Job drawing, mm, ordinate dimensions from the low corner. One solid piece. A direction names the side the tool comes from. Round coordinates to 2 decimals unless told otherwise and drop trailing zeros. Loops run counter-clockwise (first coordinate to the right, second up) from the corner with the lowest first, then second, coordinate; pieces in that order, holes last. Notation, with made-up numbers: M 15,-24.75 L 37,-24.75 A28 cw 37,-4.75 Z; hole C -15.5,72.25 d4. An arc over 180 degrees is marked long. Use a Markdown table: item, result. Add a question column.
(1) Band-saw the part on C-C, the plane z = 72. Write the cut outline in (x, y).
(2) Which spindle directions (+Z, -Z, +X, -X, +Y, -Y) get a long thin tool onto all of the face, cutting with end or side? Do the marked faces 4, 5 and 6. Say none if no direction does.
(3) Band-saw the part on A-A, the plane y = 54. Write the cut outline in (x, z).
(4) Wall check: L1, parallel to X at y = 68, z = 65.5; L2, parallel to Z at x = 92, y = 300; L3, parallel to Z at x = 51, y = 324.5. Give the ranges that are in metal, low to high.
(5) Flat gauge pins, fed straight in: P1, Ø6, axis at x = 17.98, y = 371.39, coming from the +Z side; P2, Ø14, axis at y = 86.03, z = 97.12, coming from the +X side; P3, Ø22.5, axis at x = 81, y = 350, coming from the -Z side; P4, Ø9.5, axis at y = 321.39, z = 383.02, coming from the -X side. Where does each tip first touch, or does it go through?
(6) Two-plate mould, pull along Z, no slides. Class the marked faces 1, 2 and 3: released by +Z, released by -Z, zero draft, split by the parting line, or undercut.
(7) Band-saw the part on B-B, the plane x = 39.5. Write the cut outline in (y, z).
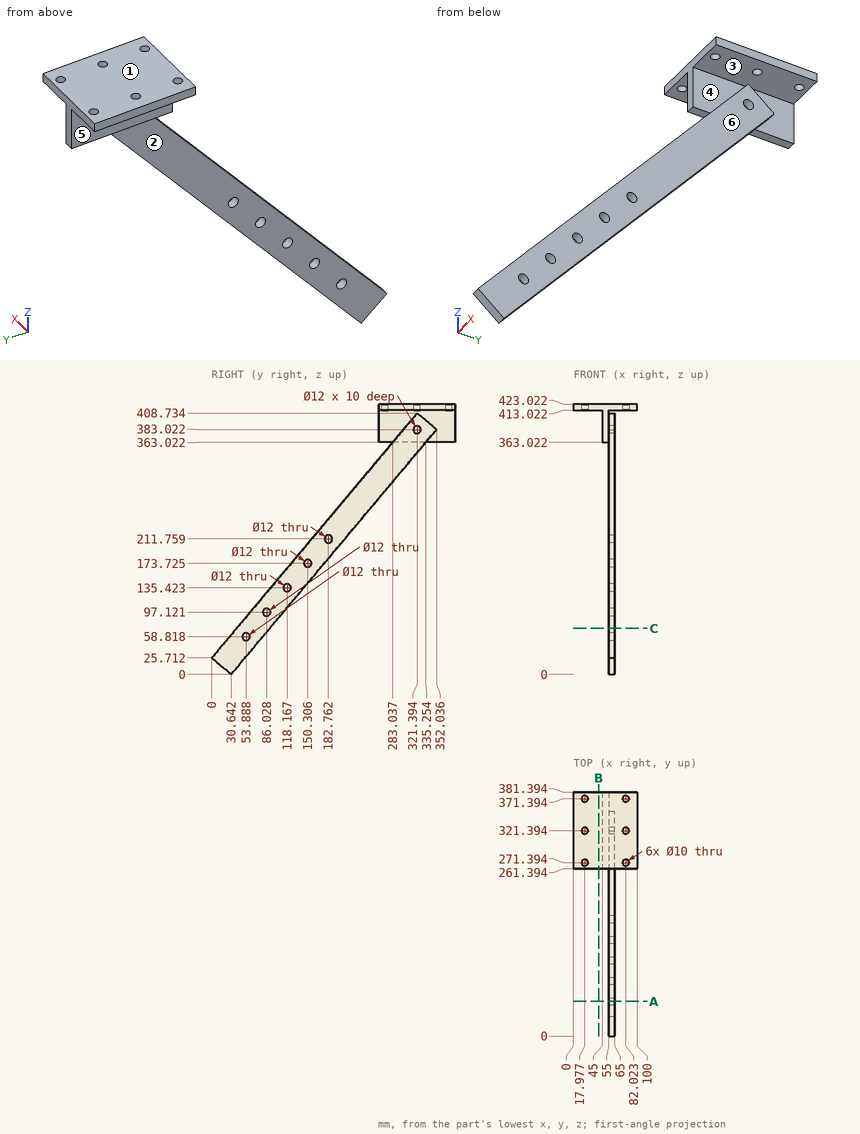
Return value:
| question | item | result |
|---|---|---|
| 1 | outline | M 55,38.84 L 65,38.84 L 65,91.06 L 55,91.06 Z |
| 2 | face 4 | +X |
| 2 | face 5 | -Z, -X, +Y, -Y |
| 2 | face 6 | -Z, +X, +Y, -Y |
| 3 | outline | M 55,27.84 L 65,27.84 L 65,52.82 L 55,52.82 Z; M 55,64.82 L 65,64.82 L 65,90.07 L 55,90.07 Z |
| 4 | L1 | 55 to 65 |
| 4 | L2 | 413.02 to 423.02 |
| 4 | L3 | 363.02 to 423.02 |
| 5 | P1 | through |
| 5 | P2 | x = 65 |
| 5 | P3 | z = 413.02 |
| 5 | P4 | x = 45 |
| 6 | face 1 | released by +Z |
| 6 | face 2 | zero draft |
| 6 | face 3 | undercut |
| 7 | outline | M 261.39,413.02 L 381.39,413.02 L 381.39,423.02 L 261.39,423.02 Z |
